Can you work these out from the model? Positions are in its coordinate system, mm. Face numbers are marked on the shaded views. A direction names the side the tool comes from. Round coordinates to 2 decimals unless told otherwise and drop trailing zeros. Order: outer loops, then holes, each group sorted by start corner. A loop starts at its lowest first (then second) coordinate and runs counter-clockwise, first axis right, second up. Notation, with made-up numbers: (41, 28) -> (89, 28) arc R14 ccw to (89, 51) -> close; hole circle Ø11 at (-19, 54.5). An arc over 180 degrees is marked (long way). Use a Markdown table: item, result. Add a question column.
Q1. We'd pull the mould along Y, two halves only. Please class the marked faces 4, 5 and 6: +Y half, -Y half, draft (parallel to the pull), parting line (faces both ways), or undercut.
Q2. If we section it at A-A on x = 0: List the corners of the cut face in (y, z) for me, plus the area to 3 significant figures.
Q3. I need wall thicknesses on line 1 along Y through (x, z) = (0, 4); line 2 along Y through (x, z) = (0, 10.75); line 3 along Z through (x, y) = (-6.75, -6.25). Which ranges of each line are inside material? Lowest first, please. Write a range as [from, to].
Q4. For the marked faces 1, 2 and 3, which set-ups out of +Z, -Z, +X, -X, +Y, -Y let a thin tool reach every point of the face, with its end or its side?
Q5. If we section it at C-C on z = 13: List the corners of the cut face in (x, y) for me, plus the area to 3 significant figures.
Q6. I'm going to push flat-ended pins straight in: pin 1 Ø2 at (x, z) = (2, 12) entering from +Y; pin 2 Ø2 at (x, z) = (6, 3.5) entering from -Y (3 decimals); pin 3 Ø2 at (x, z) = (-1.5, 13.5) entering from +Y; pin 4 Ø3 at (x, y) = (0, 0) entering from -Z. Where does each tip first touch, or does it pass through?
Q7. If we section it at D-D on y = -3.75: List the corners of the cut face in (x, z) for me, plus the area to 3 significant figures.
```python
from build123d import *

# Parameters (mm, degrees)
ESQUISSE1_R             = 10
BOSS_EXTRU_1_DEPTH      = 10
ESQUISSE2_R             = 5
BOSS_EXTRU_2_DEPTH      = 5
ESQUISSE3_R             = 2.5
ENL_V_MAT_EXTRU_1_DEPTH = 16
ESQUISSE4_W             = 8
ESQUISSE4_H             = 2


with BuildPart() as part:
    # Esquisse1 → Boss.-Extru.1 (new body)
    with BuildSketch(Plane.XY):
        Circle(ESQUISSE1_R)
    extrude(amount=BOSS_EXTRU_1_DEPTH)

    # Esquisse2 → Boss.-Extru.2 (add)
    with BuildSketch(Plane.XY.offset(10)):
        Circle(ESQUISSE2_R)
    extrude(amount=BOSS_EXTRU_2_DEPTH)

    # Esquisse3 → Enlèv. mat.-Extru.1 (cut, through all)
    with BuildSketch(Plane.XY.offset(15)):
        Circle(ESQUISSE3_R)
    extrude(amount=-ENL_V_MAT_EXTRU_1_DEPTH, mode=Mode.SUBTRACT)

    # Esquisse4 → Enlèvement de matière-Révolution1 (revolve, cut)
    with BuildSketch(Plane(origin=(0, 0, 0), x_dir=(0, 0, -1), z_dir=(1, 0, 0))):
        with Locations((-5, 9)):
            Rectangle(ESQUISSE4_W, ESQUISSE4_H)
    revolve(axis=Axis((0, 0, 0), (0, 0, 1)), mode=Mode.SUBTRACT)


solid = part.part
```
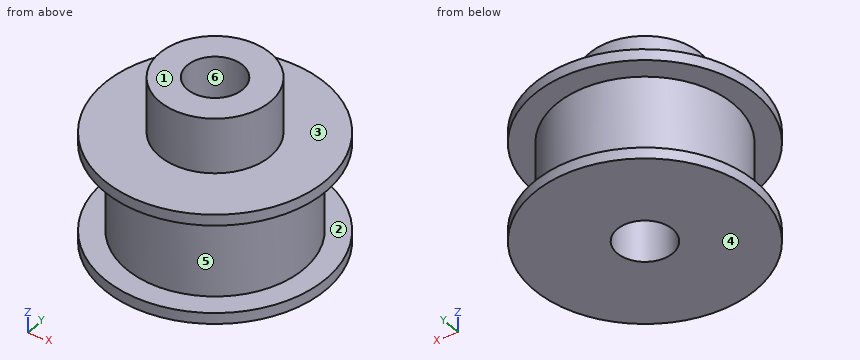
Answer below:
| question | item | result |
|---|---|---|
| 1 | face 4 | draft |
| 1 | face 5 | parting line |
| 1 | face 6 | undercut |
| 2 | outline | (-10, 0) -> (-2.5, 0) -> (-2.5, 15) -> (-5, 15) -> (-5, 10) -> (-10, 10) -> (-10, 9) -> (-8, 9) -> (-8, 1) -> (-10, 1) -> close; (2.5, 0) -> (10, 0) -> (10, 1) -> (8, 1) -> (8, 9) -> (10, 9) -> (10, 10) -> (5, 10) -> (5, 15) -> (2.5, 15) -> close |
| 2 | area | 143 mm² |
| 3 | line 1 | [-8, -2.5], [2.5, 8] |
| 3 | line 2 | [-5, -2.5], [2.5, 5] |
| 3 | line 3 | [0, 1], [9, 10] |
| 4 | face 1 | +Z, +X, -X, +Y, -Y |
| 4 | face 2 | none |
| 4 | face 3 | +Z |
| 5 | outline | circle Ø10 at (0, 0); hole circle Ø5 at (0, 0) |
| 5 | area | 58.9 mm² |
| 6 | pin 1 | y = 4.9 |
| 6 | pin 2 | y = -6.245 |
| 6 | pin 3 | y = 4.97 |
| 6 | pin 4 | through |
| 7 | outline | (-9.27, 0) -> (9.27, 0) -> (9.27, 1) -> (7.07, 1) -> (7.07, 9) -> (9.27, 9) -> (9.27, 10) -> (3.31, 10) -> (3.31, 15) -> (-3.31, 15) -> (-3.31, 10) -> (-9.27, 10) -> (-9.27, 9) -> (-7.07, 9) -> (-7.07, 1) -> (-9.27, 1) -> close |
| 7 | area | 183 mm² |
